```python
from build123d import *

# Parameters (mm, degrees)
SKETCH_9_W                 = 160
SKETCH_9_H                 = 250
EXTRUDE_499_DEPTH          = 35
SKETCH_14_W                = 160
SKETCH_14_H                = 10
CUT_EXTRUDE_746_DEPTH      = 3
HOLE_WIZARD_M6_D           = 6.6
HOLE_WIZARD_M6_CSINK_D     = 12.6
HOLE_WIZARD_M6_CSINK_ANGLE = 90
SKETCH_11_W                = 60
SKETCH_11_H                = 250
CUT_EXTRUDE_2132_DEPTH     = 24
SKETCH_15_W                = 15
SKETCH_15_H                = 300
CUT_EXTRUDE_2595_DEPTH     = 3
HOLE_WIZARD_M6_2_D         = 5
HOLE_WIZARD_3653_D         = 5


with BuildPart() as part:
    # Эскиз9 → Extrude 499 (new body)
    with BuildSketch(Plane(origin=(-20, 0, 0), x_dir=(-1, 0, 0), z_dir=(0, 0, -1))):
        with Locations((-20, 77)):
            Rectangle(SKETCH_9_W, SKETCH_9_H)
    extrude(amount=EXTRUDE_499_DEPTH)

    # Эскиз14 → Cut-Extrude 746 (cut)
    with BuildSketch(Plane(origin=(0, 0, -35), x_dir=(-1, 0, 0), z_dir=(0, 0, -1))):
        with Locations((0, 53)):
            Rectangle(SKETCH_14_W, SKETCH_14_H)
    extrude(amount=-CUT_EXTRUDE_746_DEPTH, mode=Mode.SUBTRACT)

    # Hole Wizard M6 (through all)
    with Locations(Plane.XY):
        with Locations((-40, 53), (40, 53), (-40, 16.5), (40, 16.5)):
            CounterSinkHole(HOLE_WIZARD_M6_D / 2, HOLE_WIZARD_M6_CSINK_D / 2, counter_sink_angle=HOLE_WIZARD_M6_CSINK_ANGLE)

    # Эскиз11 → Cut-Extrude 2132 (cut)
    with BuildSketch(Plane(origin=(0, 0, 0), x_dir=(-1, 0, 0), z_dir=(0, 0, -1))):
        with Locations((0, 77)):
            Rectangle(SKETCH_11_W, SKETCH_11_H)
    extrude(amount=CUT_EXTRUDE_2132_DEPTH, mode=Mode.SUBTRACT)

    # Эскиз15 → Cut-Extrude 2595 (cut)
    with BuildSketch(Plane.XY):
        with Locations((-55, 102)):
            Rectangle(SKETCH_15_W, SKETCH_15_H)
        with Locations((55, 102)):
            Rectangle(SKETCH_15_W, SKETCH_15_H)
    extrude(amount=-CUT_EXTRUDE_2595_DEPTH, mode=Mode.SUBTRACT)

    # Hole Wizard M6 2 (through all)
    with Locations(Plane.XY.offset(-24)):
        with Locations((-23, -38), (23, -38)):
            Hole(HOLE_WIZARD_M6_2_D / 2)

    # Hole Wizard 3653 (through all)
    with Locations(Plane.XY.offset(-24)):
        with Locations((-23, 162), (23, 162), (-23, 175), (23, 175)):
            Hole(HOLE_WIZARD_3653_D / 2)


solid = part.part
```
Geometry: final body of the model. Coordinates: model frame, mm. A direction names the side the tool comes from. Round coordinates to 2 decimals unless told otherwise and drop trailing zeros. Write each loop counter-clockwise with the first axis right and the second up, starting at its lowest first coordinate (ties: lowest second). Pieces come first, ordered by that corner, then holes. Notation, with made-up numbers: (-37, 66) -> (8, 66) arc R35 ccw to (8, 98) -> close; hole circle Ø5 at (-16, -37). An arc over 180 degrees is marked (long way). Return JSON: item names as keys, results as strings.
Q1. Section D-D on y = 108. Return the cut outline in (x, z).
From the geometry:
{"outline": "(-80, -35) -> (80, -35) -> (80, 0) -> (62.5, 0) -> (62.5, -3) -> (47.5, -3) -> (47.5, 0) -> (30, 0) -> (30, -24) -> (-30, -24) -> (-30, 0) -> (-47.5, 0) -> (-47.5, -3) -> (-62.5, -3) -> (-62.5, 0) -> (-80, 0) -> close"}
Q2. Ray query, line 1 (Y direction, x = -23, z = -27); line 2 (Y direction, x = 40, z = -17); line 3 (X direction, y = 16.5, z = -21.5). Return the intervals inside material, ascending.
From the geometry:
{"line 1": "-48 to -40.5, -35.5 to 159.5, 164.5 to 172.5, 177.5 to 202", "line 2": "-48 to 13.2, 19.8 to 49.7, 56.3 to 202", "line 3": "-80 to -43.3, -36.7 to -30, 30 to 36.7, 43.3 to 80"}
Q3. Set-up query: faces 1 (the conical face through (36.71, 54.03, -2.85)), 2 (the flat face through (55, 79, -3)). Return all of +Z, -Z, +X, -X, +Y, -Y with unobstructed straight access to the full face (end or side cutting, diameter ignored); none if empty.
From the geometry:
{"face 1": "+Z", "face 2": "+Z, +Y, -Y"}
Q4. Section B-B on x = 23. Return the cut outline in (y, z), and give its area (4 significant figures).
From the geometry:
{"outline": "(-48, -35) -> (-40.5, -35) -> (-40.5, -24) -> (-48, -24) -> close; (-35.5, -35) -> (48, -35) -> (48, -32) -> (58, -32) -> (58, -35) -> (159.5, -35) -> (159.5, -24) -> (-35.5, -24) -> close; (164.5, -35) -> (172.5, -35) -> (172.5, -24) -> (164.5, -24) -> close; (177.5, -35) -> (202, -35) -> (202, -24) -> (177.5, -24) -> close", "area": "2,555 mm2"}
Q5. Section A-A on y = -38. Return the cut outline in (x, z), and give its area (3 significant figures).
From the geometry:
{"outline": "(-80, -35) -> (-25.5, -35) -> (-25.5, -24) -> (-30, -24) -> (-30, 0) -> (-47.5, 0) -> (-47.5, -3) -> (-62.5, -3) -> (-62.5, 0) -> (-80, 0) -> close; (-20.5, -35) -> (20.5, -35) -> (20.5, -24) -> (-20.5, -24) -> close; (25.5, -35) -> (80, -35) -> (80, 0) -> (62.5, 0) -> (62.5, -3) -> (47.5, -3) -> (47.5, 0) -> (30, 0) -> (30, -24) -> (25.5, -24) -> close", "area": "3,960 mm2"}
Q6. Section C-C on x = -40. Return the cut outline in (y, z).
From the geometry:
{"outline": "(-48, -35) -> (13.2, -35) -> (13.2, -3) -> (10.2, 0) -> (-48, 0) -> close; (19.8, -35) -> (48, -35) -> (48, -32) -> (49.7, -32) -> (49.7, -3) -> (46.7, 0) -> (22.8, 0) -> (19.8, -3) -> close; (56.3, -32) -> (58, -32) -> (58, -35) -> (202, -35) -> (202, 0) -> (59.3, 0) -> (56.3, -3) -> close"}
Q7. Mould query, pull axis Y, two halves, no side actions, for faces 3 (the cylindrical face through (-22.46, -40.44, -29.58)), 4 (the flat face through (1, -48, -25)), 5 (the flat face through (-55, 79, -3)), 6 (the cylindrical face through (-39.57, 56.27, -17.7)). Classes: +Y half, -Y half, draft (parallel to the pull), parting line (faces both ways), or undercut.
From the geometry:
{"face 3": "undercut", "face 4": "-Y half", "face 5": "draft", "face 6": "undercut"}
Q8. First-contact query: pin 1 Ø3 at (x, y) = (-25, 174) entering from +Z; pin 2 Ø4.5 at (x, y) = (-52, 56.5) entering from +Z; pin 3 Ø8.5 at (x, y) = (-40, 53) entering from +Z; pin 4 Ø8.5 at (x, y) = (-40, 16.5) entering from -Z. Flat tips, straight axial feed; report the tip coordinate or a pass-through.
From the geometry:
{"pin 1": "z = -24", "pin 2": "z = -3", "pin 3": "z = -2.05", "pin 4": "z = -35"}
